from build123d import *

# Parameters (mm, degrees)
IZIM2_R                     = 17.5
Y_KSEKLIK_EKSTR_ZYON1_DEPTH = 45
IZIM3_R                     = 6.5
Y_KSEKLIK_EKSTR_ZYON2_DEPTH = 4
RADYUS1_R                   = 2
RADYUS2_R                   = 1
IZIM4_R                     = 1
KES_EKSTR_ZYON1_DEPTH       = 45
IZIM5_R                     = 16.5
KES_EKSTR_ZYON2_DEPTH       = 44
RADYUS3_R                   = 1
KES_EKSTR_ZYON3_DEPTH       = 44
DAIRESEL_KAPLAMA1_COUNT     = 4
IZIM9_R                     = 4.5
KES_EKSTR_ZYON4_DEPTH       = 0.5
IZIM10_R                    = 1.5
KES_EKSTR_ZYON6_DEPTH       = 30


with BuildPart() as part:
    # Çizim2 → Yükseklik-Ekstrüzyon1 (new body)
    with BuildSketch(Plane.XY):
        with Locations(Location((0, 0, 0), (0, 0, 180))):
            Circle(IZIM2_R)
    extrude(amount=Y_KSEKLIK_EKSTR_ZYON1_DEPTH)

    # Çizim3 → Yükseklik-Ekstrüzyon2 (add)
    with BuildSketch(Plane.XY.offset(45)):
        Circle(IZIM3_R)
    extrude(amount=Y_KSEKLIK_EKSTR_ZYON2_DEPTH)

    # Radyus1
    radyus1_edges = [part.edges().sort_by_distance(p)[0] for p in [
        (17.5, 0, 45),
    ]]
    fillet(radyus1_edges, radius=RADYUS1_R)

    # Radyus2
    radyus2_edges = [part.edges().sort_by_distance(p)[0] for p in [
        (-6.5, 0, 49),
    ]]
    fillet(radyus2_edges, radius=RADYUS2_R)

    # Çizim4 → Kes-Ekstrüzyon1 (cut)
    with BuildSketch(Plane.XY.offset(45)):
        with Locations((0, 12.5)):
            Circle(IZIM4_R)
    kes_ekstr_zyon1 = extrude(amount=-KES_EKSTR_ZYON1_DEPTH, mode=Mode.SUBTRACT)

    # Çizim5 → Kes-Ekstrüzyon2 (cut)
    with BuildSketch(Plane(origin=(0, 0, 0), x_dir=(-1, 0, 0), z_dir=(0, 0, -1))):
        Circle(IZIM5_R)
    extrude(amount=-KES_EKSTR_ZYON2_DEPTH, mode=Mode.SUBTRACT)

    # Radyus3
    radyus3_edges = [part.edges().sort_by_distance(p)[0] for p in [
        (16.5, 0, 44),
    ]]
    fillet(radyus3_edges, radius=RADYUS3_R)

    # Aynalama1: Kes-Ekstrüzyon1 across plane
    add(kes_ekstr_zyon1.mirror(Plane.ZX), mode=Mode.SUBTRACT)

    # Çizim7 → Kes-Ekstrüzyon3 (cut)
    with BuildSketch(Plane.XY.offset(45)):
        with BuildLine():
            ThreePointArc((8.577055255, 4.084620319), (9.100972079, 3.589155465), (9.82192332, 3.574887732))
            Line((9.82192332, 3.574887732), (10.765531412, 3.91833299))
            ThreePointArc((10.765531412, 3.91833299), (11.347352532, 4.475249801), (11.329903553, 5.28046262))
            ThreePointArc((11.329903553, 5.28046262), (8.838834765, 8.838834765), (5.28046262, 11.329903553))
            ThreePointArc((5.28046262, 11.329903553), (4.475249801, 11.347352532), (3.91833299, 10.765531412))
            Line((3.91833299, 10.765531412), (3.574887732, 9.82192332))
            ThreePointArc((3.574887732, 9.82192332), (3.589155465, 9.100972079), (4.084620319, 8.577055255))
            ThreePointArc((4.084620319, 8.577055255), (6.717514421, 6.717514421), (8.577055255, 4.084620319))
        make_face()
    kes_ekstr_zyon3 = extrude(amount=-KES_EKSTR_ZYON3_DEPTH, mode=Mode.SUBTRACT)

    # Dairesel Kaplama1: Kes-Ekstrüzyon3 ×4 about axis
    dairesel_kaplama1_axis = Axis((0, 0, 0), (0, 0, 1))
    for i in range(1, DAIRESEL_KAPLAMA1_COUNT):
        add(kes_ekstr_zyon3.rotate(dairesel_kaplama1_axis, i * 360 / DAIRESEL_KAPLAMA1_COUNT), mode=Mode.SUBTRACT)

    # Çizim9 → Kes-Ekstrüzyon4 (cut)
    with BuildSketch(Plane.XY.offset(49)):
        Circle(IZIM9_R)
    extrude(amount=-KES_EKSTR_ZYON4_DEPTH, mode=Mode.SUBTRACT)

    # Çizim10 → Kes-Ekstrüzyon6 (cut)
    with BuildSketch(Plane.XY.offset(48.5)):
        Circle(IZIM10_R)
    extrude(amount=-KES_EKSTR_ZYON6_DEPTH, mode=Mode.SUBTRACT)


solid = part.part
Design review of the part built by this model. Coordinates are the model's own, in mm. A direction names the side the tool comes from. Coordinates: 2 decimals unless noted, no trailing zeros. Loops run counter-clockwise (first coordinate to the right, second up) from the corner with the lowest first, then second, coordinate; pieces in that order, holes last.
Item 1: For faces 4 (the flat face through (-5, 0, 49)), 5 (the cylindrical face through (-0.59, 4.46, 48.75)), 6 (the cylindrical face through (-6.685, -6.75, 44.507)), 7 (the cylindrical face through (-15.24, -6.32, 21.2)), list the 3-axis set-ups (+Z, -Z, +X, -X, +Y, -Y) from which the entire face can be reached by the end or side of a thin tool; tool diameter is ignored.
Completed:
face 4: +Z, +X, -X, +Y, -Y
face 5: +Z
face 6: +Z, -Z
face 7: -Z
Item 2: Add section B-B (x = 0). Give the number of separate pieces and of enclosed holes in the cut face, and give its area (3 significant figures).
Completed:
separate pieces: 4
enclosed holes: 0
area: 151 mm2
Item 3: Add section C-C (z = 5.5). Write out the cut boundary in (x, y).
Completed:
outline: circle Ø35 at (0, 0); hole circle Ø33 at (0, 0)
Item 4: Draft analysis for pull direction X (two halves, no side actions). For faces 1 (the cylindrical face through (-8.88, -8.8, 44.51)), 2 (the flat face through (5, -16, 0)), 3 (the cylindrical face through (3.794, 17.084, 21.199)), state which applies: pulls with the +X half, pulls with the -X half, needs draft (parallel to the pull), parting line crosses it, or undercut.
Completed:
face 1: undercut
face 2: needs draft
face 3: parting line crosses it
Item 5: Add section A-A (y = 0). Write out the cut boundary in (x, z).
Completed:
outline: (-17.5, 0) - (-16.5, 0) - (-16.5, 43) arc R1 cw to (-15.5, 44) - (-1.5, 44) - (-1.5, 48.5) - (-4.5, 48.5) - (-4.5, 49) - (-5.5, 49) arc R1 ccw to (-6.5, 48) - (-6.5, 45) - (-15.5, 45) arc R2 ccw to (-17.5, 43) - close; (1.5, 44) - (15.5, 44) arc R1 cw to (16.5, 43) - (16.5, 0) - (17.5, 0) - (17.5, 43) arc R2 ccw to (15.5, 45) - (6.5, 45) - (6.5, 48) arc R1 ccw to (5.5, 49) - (4.5, 49) - (4.5, 48.5) - (1.5, 48.5) - close
Item 6: Wall thickness on L1, parallel to X at y = -12.5, z = 44.4; L2, parallel to Y at x = 0, z = 15; L3, parallel to Y at x = 0, z = 48: over which ranges is each line inside the solid? List them lowest first.
Completed:
L1: x = -11.42 to -1, 1 to 11.42
L2: y = -17.5 to -16.5, 16.5 to 17.5
L3: y = -6.5 to -1.5, 1.5 to 6.5
Item 7: Clearance check with flat-ended pins moving along their axes: pin 1 (12 mm diameter, centred on x = -11.5, z = 35, fed in from +Y); pin 2 (3 mm diameter, centred on x = 0, y = 12.5, fed in from +Z); pin 3 (10 mm diameter, centred on y = -10.5, z = 22.5, fed in from +X). State where each tip first meets the part, or that it passes through.
Completed:
pin 1: stops at y = 16.61
pin 2: stops at z = 45
pin 3: stops at x = 16.61
